from build123d import *

# Parameters (mm, degrees)
SKETCH_1_W          = 70
SKETCH_1_H          = 110
EXTRUDE_1_DEPTH     = 5
EXTRUDE_2_DEPTH     = 70
CUT_EXTRUDE_1_DEPTH = 70
SKETCH_4_W          = 12.81
SKETCH_4_H          = 10
EXTRUDE_3_DEPTH     = 70
SKETCH_5_W          = 10
SKETCH_5_H          = 15
CUT_EXTRUDE_2_DEPTH = 70
CUT_EXTRUDE_3_REACH = 124.474
SKETCH_6_R          = 11.2
SKETCH_7_R          = 1.5
CUT_EXTRUDE_4_DEPTH = 10
EXTRUDE_4_DEPTH     = 20
SKETCH_9_R          = 1.5
CUT_EXTRUDE_5_DEPTH = 10
CUT_EXTRUDE_6_REACH = 124.984
SKETCH_10_R         = 1.5
SKETCH_11_R         = 3
CUT_EXTRUDE_7_DEPTH = 3
CUT_EXTRUDE_8_REACH = 124.984
SKETCH_12_R         = 1
FILLET_1_R          = 4
SKETCH_13_R         = 1.5
CUT_EXTRUDE_9_DEPTH = 10


with BuildPart() as part:
    # 草图1 → 凸台-拉伸1 (new body)
    with BuildSketch(Plane(origin=(0, 0, 0), x_dir=(1, 0, 0), z_dir=(0, 1, 0))):
        with Locations((35, 55)):
            Rectangle(SKETCH_1_W, SKETCH_1_H)
    extrude(amount=EXTRUDE_1_DEPTH)

    # 草图2 → 凸台-拉伸2 (add)
    with BuildSketch(Plane.ZY):
        with BuildLine():
            Line((-110, -13.499982039), (-100.81, -13.499982039))
            ThreePointArc((-100.81, -13.499982039), (-89.81, -2.499982039), (-78.81, -13.499982039))
            ThreePointArc((-78.81, -13.499982039), (-67.81, -2.499982039), (-56.81, -13.499982039))
            ThreePointArc((-56.81, -13.499982039), (-45.81, -2.499982039), (-34.81, -13.499982039))
            ThreePointArc((-34.81, -13.499982039), (-23.81, -2.499982039), (-12.81, -13.499982039))
            Line((-12.81, -13.499982039), (-12.81, 0))
            Line((-12.81, 0), (-110, 0))
            Line((-110, 0), (-110, -13.499982039))
        make_face()
    extrude(amount=-EXTRUDE_2_DEPTH)

    # 草图3 → 切除-拉伸1 (cut)
    with BuildSketch(Plane.ZY):
        with BuildLine():
            Line((-100.238332835, -10), (-110, -10))
            Line((-110, -10), (-110, -13.499982039))
            Line((-110, -13.499982039), (-100.81, -13.499982039))
            ThreePointArc((-100.81, -13.499982039), (-100.666142528, -11.726801449), (-100.238332835, -10))
        make_face()
        with BuildLine():
            Line((-78.238332835, -10), (-79.381667165, -10))
            ThreePointArc((-79.381667165, -10), (-78.953857472, -11.726801449), (-78.81, -13.499982039))
            ThreePointArc((-78.81, -13.499982039), (-78.666142528, -11.726801449), (-78.238332835, -10))
        make_face()
        with BuildLine():
            Line((-56.238332835, -10), (-57.381667165, -10))
            ThreePointArc((-57.381667165, -10), (-56.953857472, -11.726801449), (-56.81, -13.499982039))
            ThreePointArc((-56.81, -13.499982039), (-56.666142528, -11.726801449), (-56.238332835, -10))
        make_face()
        with BuildLine():
            Line((-12.81, -13.499982039), (-12.81, -10))
            Line((-12.81, -10), (-13.381667165, -10))
            ThreePointArc((-13.381667165, -10), (-12.953857472, -11.726801449), (-12.81, -13.499982039))
        make_face()
        with BuildLine():
            Line((-34.238332835, -10), (-35.381667165, -10))
            ThreePointArc((-35.381667165, -10), (-34.953857472, -11.726801449), (-34.81, -13.499982039))
            ThreePointArc((-34.81, -13.499982039), (-34.666142528, -11.726801449), (-34.238332835, -10))
        make_face()
    extrude(amount=-CUT_EXTRUDE_1_DEPTH, mode=Mode.SUBTRACT)

    # 草图4 → 凸台-拉伸3 (add)
    with BuildSketch(Plane.ZY):
        with Locations((-6.405, -5)):
            Rectangle(SKETCH_4_W, SKETCH_4_H)
    extrude(amount=-EXTRUDE_3_DEPTH)

    # 草图5 → 切除-拉伸2 (cut)
    with BuildSketch(Plane.ZY):
        with Locations((-105, -2.5)):
            Rectangle(SKETCH_5_W, SKETCH_5_H)
    extrude(amount=-CUT_EXTRUDE_2_DEPTH, mode=Mode.SUBTRACT)

    # 草图6 → 切除-拉伸3 (cut, up to next)
    with BuildSketch(Plane.ZY, mode=Mode.PRIVATE) as cut_extrude_3_sk1:
        with Locations((-89.81, -13.499982039)):
            Circle(SKETCH_6_R)
    cut_extrude_3_tool1 = extrude(cut_extrude_3_sk1.sketch, amount=-CUT_EXTRUDE_3_REACH, mode=Mode.PRIVATE) & part.part
    # 草图6 → 切除-拉伸3 (cut, up to next)
    with BuildSketch(Plane.ZY, mode=Mode.PRIVATE) as cut_extrude_3_sk2:
        with Locations((-67.81, -13.499982039)):
            Circle(SKETCH_6_R)
    cut_extrude_3_tool2 = extrude(cut_extrude_3_sk2.sketch, amount=-CUT_EXTRUDE_3_REACH, mode=Mode.PRIVATE) & part.part
    # 草图6 → 切除-拉伸3 (cut, up to next)
    with BuildSketch(Plane.ZY, mode=Mode.PRIVATE) as cut_extrude_3_sk3:
        with Locations((-45.81, -13.499982039)):
            Circle(SKETCH_6_R)
    cut_extrude_3_tool3 = extrude(cut_extrude_3_sk3.sketch, amount=-CUT_EXTRUDE_3_REACH, mode=Mode.PRIVATE) & part.part
    # 草图6 → 切除-拉伸3 (cut, up to next)
    with BuildSketch(Plane.ZY, mode=Mode.PRIVATE) as cut_extrude_3_sk4:
        with Locations((-23.81, -13.499982039)):
            Circle(SKETCH_6_R)
    cut_extrude_3_tool4 = extrude(cut_extrude_3_sk4.sketch, amount=-CUT_EXTRUDE_3_REACH, mode=Mode.PRIVATE) & part.part
    add(cut_extrude_3_tool1.solids().sort_by_distance((0, -13.499982, -89.81))[0], mode=Mode.SUBTRACT)
    add(cut_extrude_3_tool2.solids().sort_by_distance((0, -13.499982, -67.81))[0], mode=Mode.SUBTRACT)
    add(cut_extrude_3_tool3.solids().sort_by_distance((0, -13.499982, -45.81))[0], mode=Mode.SUBTRACT)
    add(cut_extrude_3_tool4.solids().sort_by_distance((0, -13.499982, -23.81))[0], mode=Mode.SUBTRACT)

    # 草图7 → 切除-拉伸4 (cut)
    with BuildSketch(Plane(origin=(70, 0, 0), x_dir=(0, 0, -1), z_dir=(1, 0, 0))):
        with Locations((78.81000898, -1)):
            Circle(SKETCH_7_R)
        with Locations((34.81000898, -1)):
            Circle(SKETCH_7_R)
    extrude(amount=-CUT_EXTRUDE_4_DEPTH, mode=Mode.SUBTRACT)

    # 草图8 → 凸台-拉伸4 (add)
    with BuildSketch(Plane.ZY):
        Polygon((0, 5), (-100, 5), (-100, -2.299982039), (-12.61, -2.299982039), (-12.61, -10), (0, -10), (0, -2.299982039), align=None)
    extrude(amount=EXTRUDE_4_DEPTH)

    # 草图9 → 切除-拉伸5 (cut)
    with BuildSketch(Plane(origin=(0, 0, -100), x_dir=(-1, 0, 0), z_dir=(0, 0, -1))):
        with Locations((-58, 1.35000898)):
            Circle(SKETCH_9_R)
        with Locations((8, 1.35000898)):
            Circle(SKETCH_9_R)
    extrude(amount=-CUT_EXTRUDE_5_DEPTH, mode=Mode.SUBTRACT)

    # 草图10 → 切除-拉伸6 (cut, up to next)
    with BuildSketch(Plane(origin=(0, 5, 0), x_dir=(1, 0, 0), z_dir=(0, 1, 0)), mode=Mode.PRIVATE) as cut_extrude_6_sk1:
        with Locations(Location((-8, 6.305, 0), (0, 0, 270))):
            Circle(SKETCH_10_R)
    cut_extrude_6_tool1 = extrude(cut_extrude_6_sk1.sketch, amount=-CUT_EXTRUDE_6_REACH, mode=Mode.PRIVATE) & part.part
    # 草图10 → 切除-拉伸6 (cut, up to next)
    with BuildSketch(Plane(origin=(0, 5, 0), x_dir=(1, 0, 0), z_dir=(0, 1, 0)), mode=Mode.PRIVATE) as cut_extrude_6_sk2:
        with Locations(Location((58, 6.305, 0), (0, 0, 270))):
            Circle(SKETCH_10_R)
    cut_extrude_6_tool2 = extrude(cut_extrude_6_sk2.sketch, amount=-CUT_EXTRUDE_6_REACH, mode=Mode.PRIVATE) & part.part
    add(cut_extrude_6_tool1.solids().sort_by_distance((-8, 5, -6.305))[0], mode=Mode.SUBTRACT)
    add(cut_extrude_6_tool2.solids().sort_by_distance((58, 5, -6.305))[0], mode=Mode.SUBTRACT)

    # 草图11 → 切除-拉伸7 (cut)
    with BuildSketch(Plane(origin=(0, 5, 0), x_dir=(1, 0, 0), z_dir=(0, 1, 0))):
        with Locations(Location((-8, 6.305, 0), (0, 0, 270))):
            Circle(SKETCH_11_R)
        with Locations(Location((58, 6.305, 0), (0, 0, 270))):
            Circle(SKETCH_11_R)
    extrude(amount=-CUT_EXTRUDE_7_DEPTH, mode=Mode.SUBTRACT)

    # 草图12 → 切除-拉伸8 (cut, up to next)
    with BuildSketch(Plane(origin=(0, 5, 0), x_dir=(1, 0, 0), z_dir=(0, 1, 0)), mode=Mode.PRIVATE) as cut_extrude_8_sk1:
        with Locations(Location((7.891, 6.943325734, 0), (0, 0, 270))):
            Circle(SKETCH_12_R)
    cut_extrude_8_tool1 = extrude(cut_extrude_8_sk1.sketch, amount=-CUT_EXTRUDE_8_REACH, mode=Mode.PRIVATE) & part.part
    add(cut_extrude_8_tool1.solids().sort_by_distance((7.891, 5, -6.943326))[0], mode=Mode.SUBTRACT)

    # 圆角1
    # the kernel refuses this fillet: 4 mm, written as the material it takes off along each edge
    with BuildSketch(Plane(origin=(80, 5, 0), x_dir=(0, -1, 0), z_dir=(-1, 0, 0))) as fillet_1_piece_1:
        with BuildLine():
            CenterArc((FILLET_1_R, -FILLET_1_R), FILLET_1_R, 90, 90)
            Line((0, -FILLET_1_R), (0, 0))
            Line((0, 0), (FILLET_1_R, 0))
        make_face()
    extrude(amount=110, mode=Mode.SUBTRACT)

    # 草图13 → 切除-拉伸9 (cut)
    with BuildSketch(Plane.ZY.offset(20)):
        with Locations((-55, 1.35000898)):
            Circle(SKETCH_13_R)
    extrude(amount=-CUT_EXTRUDE_9_DEPTH, mode=Mode.SUBTRACT)


solid = part.part
The listing builds one solid part. Answer for the finished solid, in the listing's coordinates (mm). A direction names the side the tool comes from. Coordinates: 2 decimals unless noted, no trailing zeros. Write each loop counter-clockwise with the first axis right and the second up, starting at its lowest first coordinate (ties: lowest second). Pieces come first, ordered by that corner, then holes. Notation, with made-up numbers: M -26.75,18 L -10.75,18 A5 cw -10.75,26 Z; hole C 47.25,-26 d5. An arc over 180 degrees is marked long. Put each result on its own line as item: value. Start each with the question number.
1. Which of the six approach directions +Z, -Z, +X, -X, +Y, -Y give full straight-line access (tool end or side, diameter ignored) to faces 4 (the flat face through (60, -1, -35)), 5 (the cylindrical face through (-15.07, 1.8, -53.57)), 6 (the flat face through (-10, -2.3, -57)), 7 (the flat face through (-9, 2, -8)), 8 (the flat face through (58, 1, -90))?
2. A cutting plane is placed at D-D on z = -71. Write down the section's boundary in (x, y), then the cut area to 3 significant figures.
3. A cutting plane is placed at C-C on x = -8. Write down the section's boundary in (y, z) (3 decimals).
4. A cutting plane is placed at A-A on y = -6.75. Write down the section's boundary in (x, z) (3 decimals), then the cut area to 3 significant figures.
5. Consider line 1 (Z direction, x = 43.5, y = -3.5); line 2 (X direction, y = 1, z = -92.5); line 3 (Z direction, x = 9, y = -4.5). Determine where each line is inside the solid, lowest interval first. Write a range as from..to.
6. For a pull along Z with two mould halves and no side action, classify faces 1 (the flat face through (-8, 1, -90)), 2 (the flat face through (26, -10, -7)), 3 (the flat face through (-10, 1, -55)) as pulls with the +Z half, pulls with the -Z half, needs draft (parallel to the pull), parting line crosses it, or undercut.
7. Flat-ended cylindrical pins translate along their axes: P1, Ø5, axis at y = -5.5, z = -95.5, coming from the -X side; P2, Ø12, axis at x = 59.5, z = -68.5, coming from the -Y side; P3, Ø1.8, axis at x = -8, z = -6.305, coming from the +Y side; P4, Ø1.8, axis at x = 58, y = 1.35, coming from the -Z side. Find the tip coordinate at first contact, or state that the pin passes through.
8. A cutting plane is placed at B-B on x = 14. Write down the section's boundary in (y, z).
Resolved:
1. face 4: +X
1. face 5: -X
1. face 6: -Z, -X, -Y
1. face 7: +Y
1. face 8: -Z
2. outline: M -20,-2.3 L 0,-2.3 L 0,-2.76 L 70,-2.76 L 70,5 L -20,5 Z
2. area: 689 mm2
3. outline: M -10,-12.61 L -2.3,-12.61 L -2.3,-100 L -0.15,-100 L -0.15,-90 L 2.85,-90 L 2.85,-100 L 5,-100 L 5,-9.305 L 2,-9.305 L 2,-7.805 L -10,-7.805 Z; M -10,-4.805 L 2,-4.805 L 2,-3.305 L 4.939,-3.305 A4 ccw 1,0 L -10,0 Z
4. outline: M -20,-12.61 L 0,-12.61 L 0,-14.873 L 70,-14.873 L 70,0 L -20,0 Z; M 0,-100 L 70,-100 L 70,-98.747 L 0,-98.747 Z; M 0,-80.873 L 70,-80.873 L 70,-76.747 L 0,-76.747 Z; M 0,-58.873 L 70,-58.873 L 70,-54.747 L 0,-54.747 Z; M 0,-36.873 L 70,-36.873 L 70,-32.747 L 0,-32.747 Z; hole C -8,-6.305 d3; hole C 7.891,-6.943 d2; hole C 58,-6.305 d3
4. area: 2,230 mm2
5. line 1: z = -100..-94.85, -84.77..-72.85, -62.77..-50.85, -40.77..-28.85, -18.77..0
5. line 2: x = -20..-9.46, -6.54..56.54, 59.46..70
5. line 3: z = -100..-96.48, -83.14..-74.48, -61.14..-52.48, -39.14..-30.48, -17.14..0
6. face 1: pulls with the -Z half
6. face 2: needs draft
6. face 3: undercut
7. P1: stops at x = 0
7. P2: stops at y = -4.52
7. P3: passes through
7. P4: stops at z = -90
8. outline: M -10,-79.17 A11.2 cw -8.85,-100 L 5,-100 L 5,-4 A4 ccw 1,0 L -10,0 L -10,-13.17 A11.2 cw -10,-34.45 L -10,-35.17 A11.2 cw -10,-56.45 L -10,-57.17 A11.2 cw -10,-78.45 Z
